Geometry: final body of the model. Coordinates: model frame, mm. A direction names the side the tool comes from. Coordinates: 2 decimals unless noted, no trailing zeros. Order: outer loops, then holes, each group sorted by start corner. A loop starts at its lowest first (then second) coordinate and runs counter-clockwise, first axis right, second up. Notation, with made-up numbers: (78, -27.5) -> (97, -27.5) arc R24 ccw to (97, 3.5) -> close; hole circle Ø2 at (-27, 18.25). An arc over 180 degrees is marked (long way). Use one line per item in the form item = value.
Autodesk Inventor part; units mm, degrees
ref_plane "YZ Plane" through (0, 0, 0) normal (1, 0, 0) x (0, 1, 0)
ref_plane "XZ Plane" through (0, 0, 0) normal (0, 1, 0) x (-1, 0, 0)
ref_plane "XY Plane" through (0, 0, 0) normal (0, 0, 1) x (1, 0, 0)
sketch "Skizze1" plane through (0, 0, 0) normal (0, 0, 1) x (1, 0, 0)
  circle A0 centre (0, 0) radius 10
  dimension "d0" = 20
extrude "Extrusion1" add sketch "Skizze1" along normal blind 5
sketch "Skizze2" plane through (0, 0, 5) normal (0, 0, 1) x (1, 0, 0)
  circle A0 centre (0, 0) radius 6.5
  dimension "d3" = 13
extrude "Extrusion2" add sketch "Skizze2" along normal blind 5
sketch "Skizze3" plane through (0, 0, 5) normal (0, 0, 1) x (1, 0, 0)
  circle A0 centre (0, 0) radius 6.5
  circle A1 centre (0, 0) radius 10
  line L0 (-7.5993, 6.5) -> (7.5993, 6.5)
extrude "Extrusion3" cut sketch "Skizze3" against normal through all contours L0 A1 picked at (4.4606, 7.0529)
sketch "Skizze4" plane through (0, 0, 10) normal (0, 0, 1) x (1, 0, 0)
  circle A0 centre (0, 0) radius 3
  dimension "d8" = 6
extrude "Extrusion4" add sketch "Skizze4" along normal blind 0.5
sketch "Skizze5" plane through (0, 0, 10.5) normal (0, 0, 1) x (1, 0, 0)
  point P0 (0, 0)
hole "Bohrung1" at (0, 0, 10.5) direction (0, 0, -1) diameter 4 end through all
chamfer "Fase1" distance 0.5 angle 45 1 edges at (-3, 0, 10)
properties part number "Belt_T_Spacer" material "Aluminium 6061"
1) Contact query for flat-ended pins moving along their axis: P1, Ø5, axis at y = -8, z = 8.5, coming from the -X side; P2, Ø6, axis at x = 5.5, z = 5, coming from the -Y side; P3, Ø1, axis at y = -2.5, z = 4, coming from the -X side. Output: stop coordinate, or through.
Results found:
P1 = -3.46
P2 = -9.68
P3 = -9.8
2) Material intervals for probe 1 along Y at (x, z) = (0, 7.75); probe 2 along X at (y, z) = (0, 4); probe 3 along Z at (x, y) = (0, -7), sorted ascending. Write a range as from..to.
Results found:
probe_1 = -6.5..-2, 2..6.5
probe_2 = -10..-2, 2..10
probe_3 = 0..5
3) Section C-C, the plane x = -5. Output: boundary loops of the cut face in (y, z).
Results found:
outline = (-8.66, 0) -> (6.5, 0) -> (6.5, 5) -> (4.15, 5) -> (4.15, 10) -> (-4.15, 10) -> (-4.15, 5) -> (-8.66, 5) -> close
4) Section D-D, the plane y = -6.25. Output: boundary loops of the cut face in (x, z).
Results found:
outline = (-7.81, 0) -> (7.81, 0) -> (7.81, 5) -> (1.79, 5) -> (1.79, 10) -> (-1.79, 10) -> (-1.79, 5) -> (-7.81, 5) -> close
5) Section B-B, the plane z = 5.75. Output: boundary loops of the cut face in (x, y).
Results found:
outline = circle Ø13 at (0, 0); hole circle Ø4 at (0, 0)
6) Access query for faces 1 (the cylindrical face through (0, -10, 2)), 2 (the flat face through (3, -3, 10)). Directions: +Z, -Z, +X, -X, +Y, -Y. A direction counts if a zero-diameter tool reaches every point of the face in a straight line with its end or side. Return the directions, or none.
Results found:
face_1 = +Z, -Z
face_2 = +Z
